For this review, take the finished solid that the model builds, in its own axes (mm). A direction names the side the tool comes from. Coordinates: 2 decimals unless noted, no trailing zeros. Loops run counter-clockwise (first coordinate to the right, second up) from the corner with the lowest first, then second, coordinate; pieces in that order, holes last. Notation, with made-up numbers: (42.5, 1.25) -> (82.5, 1.25) arc R28 cw to (82.5, 28.25) -> close; hole circle Ø9 at (-27.5, 41). An arc over 180 degrees is marked (long way). Answer in a Markdown table with one row per item.
from build123d import *

# Parameters (mm, degrees)
F0_W     = 35
F0_H     = 35
F0_W_2   = 12
F0_H_2   = 12
F1_DEPTH = 1
F2_DEPTH = 1.2
F3_R     = 3
F4_R     = 5
F5_R     = 3
F6_DEPTH = 25


with BuildPart() as f1:
    # F0 (on Top) → F1 (new body)
    with BuildSketch(Plane.XY):
        Rectangle(F0_W, F0_H)
        Rectangle(F0_W_2, F0_H_2, mode=Mode.SUBTRACT)
    extrude(amount=F1_DEPTH)

    # F0 (on Top) → F2 (join)
    with BuildSketch(Plane.XY):
        Rectangle(F0_W_2, F0_H_2)
    extrude(amount=F2_DEPTH)

    # F3
    f3_edges = [f1.edges().sort_by_distance(p)[0] for p in [
        (-6, -6, 1.1),
        (6, -6, 1.1),
        (6, 6, 1.1),
        (-6, 6, 1.1),
    ]]
    fillet(f3_edges, radius=F3_R)

    # F4
    f4_edges = [f1.edges().sort_by_distance(p)[0] for p in [
        (-17.5, -17.5, 0.5),
        (17.5, -17.5, 0.5),
        (17.5, 17.5, 0.5),
        (-17.5, 17.5, 0.5),
    ]]
    fillet(f4_edges, radius=F4_R)

    # F5 (on face) → F6 (cut)
    with BuildSketch(Plane.XY.offset(1.2)):
        Circle(F5_R)
    extrude(amount=-F6_DEPTH, mode=Mode.SUBTRACT)


solid = f1.part
Item 1: The part is to be moulded in two halves that separate along X. For faces 3 (the cylindrical face through (16, 16.07, 0.51)), 4 (the cylindrical face through (-3, 0, 1)), 5 (the flat face through (4, 0, 0)), 6 (the flat face through (-17.5, -0.2, 0.5)), say which applies: +X half, -X half, draft (parallel to the pull), parting line (faces both ways), or undercut.
Worked answers:
| item | result |
|---|---|
| face 3 | +X half |
| face 4 | undercut |
| face 5 | draft |
| face 6 | -X half |
Item 2: Take a section at C-C, the plane z = 0.75. State the section outline as (x, y) points.
Worked answers:
| item | result |
|---|---|
| outline | (-17.5, -12.5) arc R5 ccw to (-12.5, -17.5) -> (12.5, -17.5) arc R5 ccw to (17.5, -12.5) -> (17.5, 12.5) arc R5 ccw to (12.5, 17.5) -> (-12.5, 17.5) arc R5 ccw to (-17.5, 12.5) -> close; hole circle Ø6 at (0, 0) |
Item 3: Take a section at B-B, the plane y = -1. State the section outline as (x, z) points.
Worked answers:
| item | result |
|---|---|
| outline | (-17.5, 0) -> (-2.83, 0) -> (-2.83, 1.2) -> (-6, 1.2) -> (-6, 1) -> (-17.5, 1) -> close; (2.83, 0) -> (17.5, 0) -> (17.5, 1) -> (6, 1) -> (6, 1.2) -> (2.83, 1.2) -> close |
Item 4: For faces 1 (the flat face through (-0.2, 17.5, 0.5)), 2 (the flat face through (8, 0, 1)), list the 3-axis set-ups (+Z, -Z, +X, -X, +Y, -Y) from which the entire face can be reached by the end or side of a thin tool; tool diameter is ignored.
Worked answers:
| item | result |
|---|---|
| face 1 | +Z, -Z, +X, -X, +Y |
| face 2 | +Z |
Item 5: Take a section at A-A, the plane x = 0. State the section outline as (y, z) points.
Worked answers:
| item | result |
|---|---|
| outline | (-17.5, 0) -> (-3, 0) -> (-3, 1.2) -> (-6, 1.2) -> (-6, 1) -> (-17.5, 1) -> close; (3, 0) -> (17.5, 0) -> (17.5, 1) -> (6, 1) -> (6, 1.2) -> (3, 1.2) -> close |
Item 6: Take a section at D-D, the plane x = -3.5. State the section outline as (y, z) points, and give its area (3 significant figures).
Worked answers:
| item | result |
|---|---|
| outline | (-17.5, 0) -> (17.5, 0) -> (17.5, 1) -> (5.96, 1) -> (5.96, 1.2) -> (-5.96, 1.2) -> (-5.96, 1) -> (-17.5, 1) -> close |
| area | 37.4 mm² |
Item 7: Insertion check: pin 1 (1 mm diameter, centred on x = 0, y = -13, fed in from +Z). The pin has a flat end and moves straight along its axis. Give the tip position at first contact, or say it passes through.
Worked answers:
| item | result |
|---|---|
| pin 1 | z = 1 |
Item 8: For L1, parallel to Y at x = 0, z = 0.25; L2, parallel to Z at x = 9.5, y = -14; L3, parallel to X at y = 16.5, z = 0.35, list the stretches that pass through material, from the lowest coordinate up.
Worked answers:
| item | result |
|---|---|
| L1 | -17.5 to -3, 3 to 17.5 |
| L2 | 0 to 1 |
| L3 | -15.5 to 15.5 |
